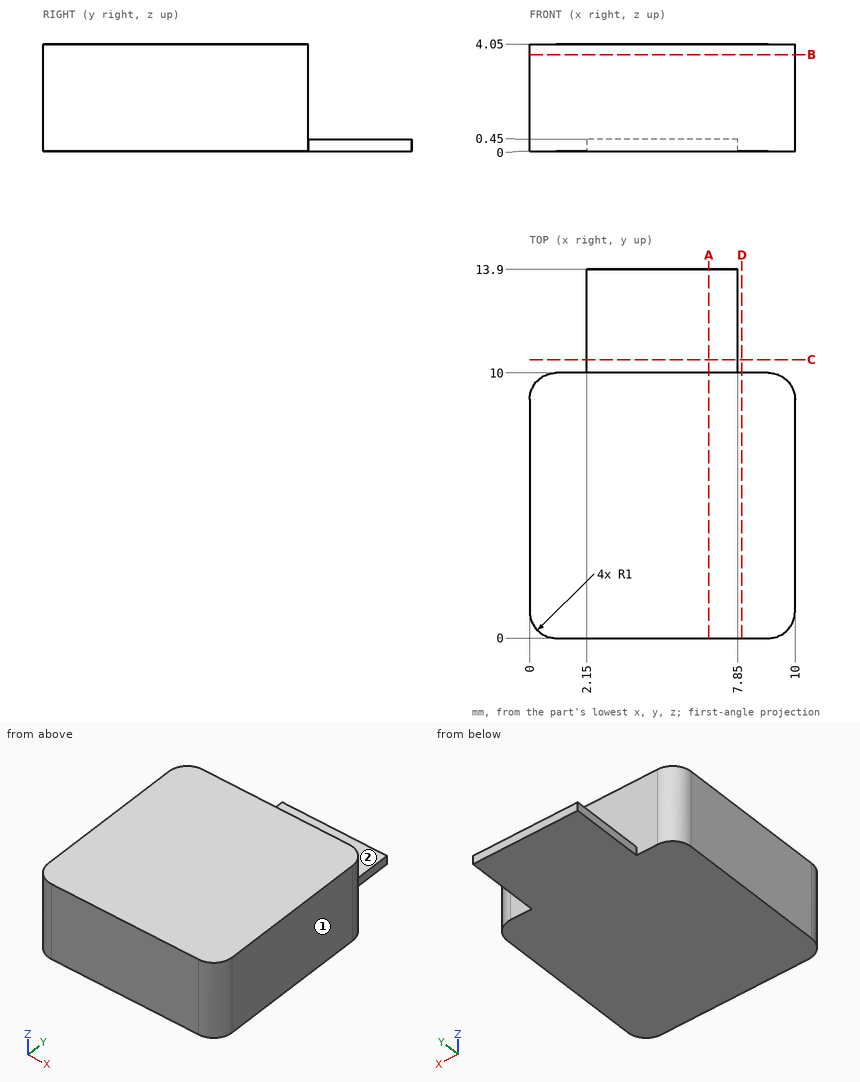
Input: dimensioned drawing with shaded views. Units: mm. Origin: part minimum x, y, z. A direction names the side the tool comes from. Coordinates: 2 decimals unless noted, no trailing zeros. Order: outer loops, then holes, each group sorted by start corner. A loop starts at its lowest first (then second) coordinate and runs counter-clockwise, first axis right, second up. Notation, with made-up numbers: (-29.75, 23.5) - (17.25, 23.5) arc R18 cw to (17.25, 30.5) - close; hole circle Ø10 at (88, 76.5). An arc over 180 degrees is marked (long way). Put each result on its own line as item: value.
1. Cut plane A-A on x = 6.75. Return the cut outline in (y, z).
Report:
outline: (0, 0) - (13.9, 0) - (13.9, 0.45) - (10, 0.45) - (10, 4.05) - (0, 4.05) - close
2. Cut plane D-D on x = 8. Return the cut outline in (y, z).
Report:
outline: (0, 0) - (10, 0) - (10, 4.05) - (0, 4.05) - close
3. Cut plane B-B on z = 3.65. Return the cut outline in (x, y), then the cut area to 3 significant figures.
Report:
outline: (0, 1) arc R1 ccw to (1, 0) - (9, 0) arc R1 ccw to (10, 1) - (10, 9) arc R1 ccw to (9, 10) - (1, 10) arc R1 ccw to (0, 9) - close
area: 99.1 mm2
4. Contact query for a flat-ended pin moving along its axis: pin 1 Ø2 at (x, z) = (4, 2) entering from +Y. Output: stop coordinate, or through.
Report:
pin 1: stops at y = 10
5. Line query: line 1 along X through (y, z) = (11, 0.4); line 2 along Y through (x, z) = (1, 2.2); line 3 along Z through (x, y) = (3.5, 10.75). Output: solid intervals per line, ascending.
Report:
line 1: x = 2.15 to 7.85
line 2: y = 0 to 10
line 3: z = 0 to 0.45
6. Cut plane C-C on y = 10.5. Return the cut outline in (x, z).
Report:
outline: (2.15, 0) - (7.85, 0) - (7.85, 0.45) - (2.15, 0.45) - close
7. Reachability of the marked faces 1 and 2 from +Z, -Z, +X, -X, +Y, -Y: full face, straight path, thin tool, end or side. Return the list, or none.
Report:
face 1: +Z, -Z, +X, +Y, -Y
face 2: +Z, +X, -X, +Y
